from build123d import *

# Parameters (mm, degrees)
SKETCH1_R           = 50.546
SKETCH1_R_2         = 4.7625
SKETCH1_W           = 25.4
SKETCH1_H           = 6.35
BOSS_EXTRUDE1_DEPTH = 6.35


with BuildPart() as part:
    # Sketch1 → Boss-Extrude1 (new body)
    with BuildSketch(Plane(origin=(0, 0, 0), x_dir=(1, 0, 0), z_dir=(0, 1, 0))):
        with Locations(Location((0, 0, 0), (0, 0, 270))):
            Circle(SKETCH1_R)
        with Locations(Location((0, 0, 0), (0, 0, 270))):
            Circle(SKETCH1_R_2, mode=Mode.SUBTRACT)
        with Locations((-25.4, 12.7)):
            Rectangle(SKETCH1_W, SKETCH1_H, mode=Mode.SUBTRACT)
        with Locations((25.4, 12.7)):
            Rectangle(SKETCH1_W, SKETCH1_H, mode=Mode.SUBTRACT)
    extrude(amount=BOSS_EXTRUDE1_DEPTH)


solid = part.part
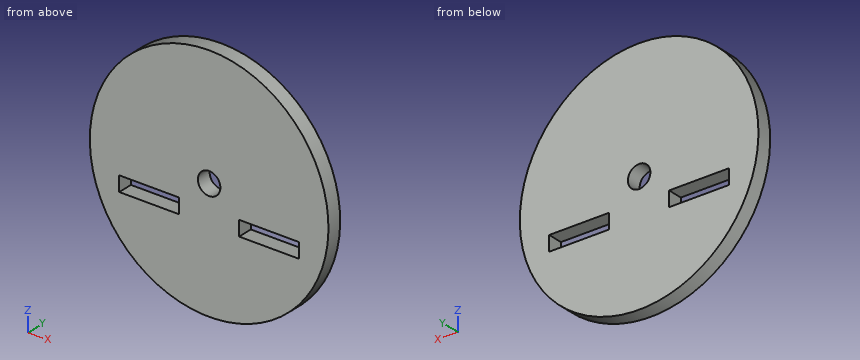
Geometry: final body of the model. Coordinates: model frame, mm. Round coordinates to 2 decimals unless told otherwise and drop trailing zeros. Loops run counter-clockwise (first coordinate to the right, second up) from the corner with the lowest first, then second, coordinate; pieces in that order, holes last.
Q1. Section B-B on x = 0. Return loops of the section in (y, z).
Q2. Material intervals for L1, parallel to X at y = 4, z = 0; L2, parallel to Z at x = 29, y = 4.25 (3 decimals); L3, parallel to Z at x = 30.5, y = 3.5 (3 decimals), sorted ascending.
Q3. Pin query (flat end, axial travel): P1, Ø7.5, axis at x = 0, z = 0, coming from the -Y side; P2, Ø1, axis at y = 5, z = 26.5, coming from the -X side; P3, Ø1.9, axis at y = 3.5, z = -12, coming from the -X side; P4, Ø3, axis at x = -23, y = 4, coming from the -Z side. Return the tip coordinate at first contact, or that it passes through.
Q4. Section C-C on y = 1. Return loops of the section in (x, z) (1 decimal).
Q5. Section A-A on z = 0. Return loops of the section in (x, y), plus the area to 3 significant figures.
Q6. Section D-D on x = 11. Return loops of the section in (y, z).
Evaluation:
1. outline: (0, -50.55) - (6.35, -50.55) - (6.35, -4.76) - (0, -4.76) - close; (0, 4.76) - (6.35, 4.76) - (6.35, 50.55) - (0, 50.55) - close
2. L1: x = -50.55 to -4.76, 4.76 to 50.55
2. L2: z = -41.399 to -15.875, -9.525 to 41.399
2. L3: z = -40.307 to -15.875, -9.525 to 40.307
3. P1: passes through
3. P2: stops at x = -43.35
3. P3: stops at x = -49.32
3. P4: stops at z = -45.75
4. outline: circle Ø101.1 at (0, 0); hole (-38.1, -15.9) - (-12.7, -15.9) - (-12.7, -9.5) - (-38.1, -9.5) - close; hole circle Ø9.5 at (0, 0); hole (12.7, -15.9) - (38.1, -15.9) - (38.1, -9.5) - (12.7, -9.5) - close
5. outline: (-50.55, 0) - (-4.76, 0) - (-4.76, 6.35) - (-50.55, 6.35) - close; (4.76, 0) - (50.55, 0) - (50.55, 6.35) - (4.76, 6.35) - close
5. area: 581 mm2
6. outline: (0, -49.33) - (6.35, -49.33) - (6.35, 49.33) - (0, 49.33) - close
